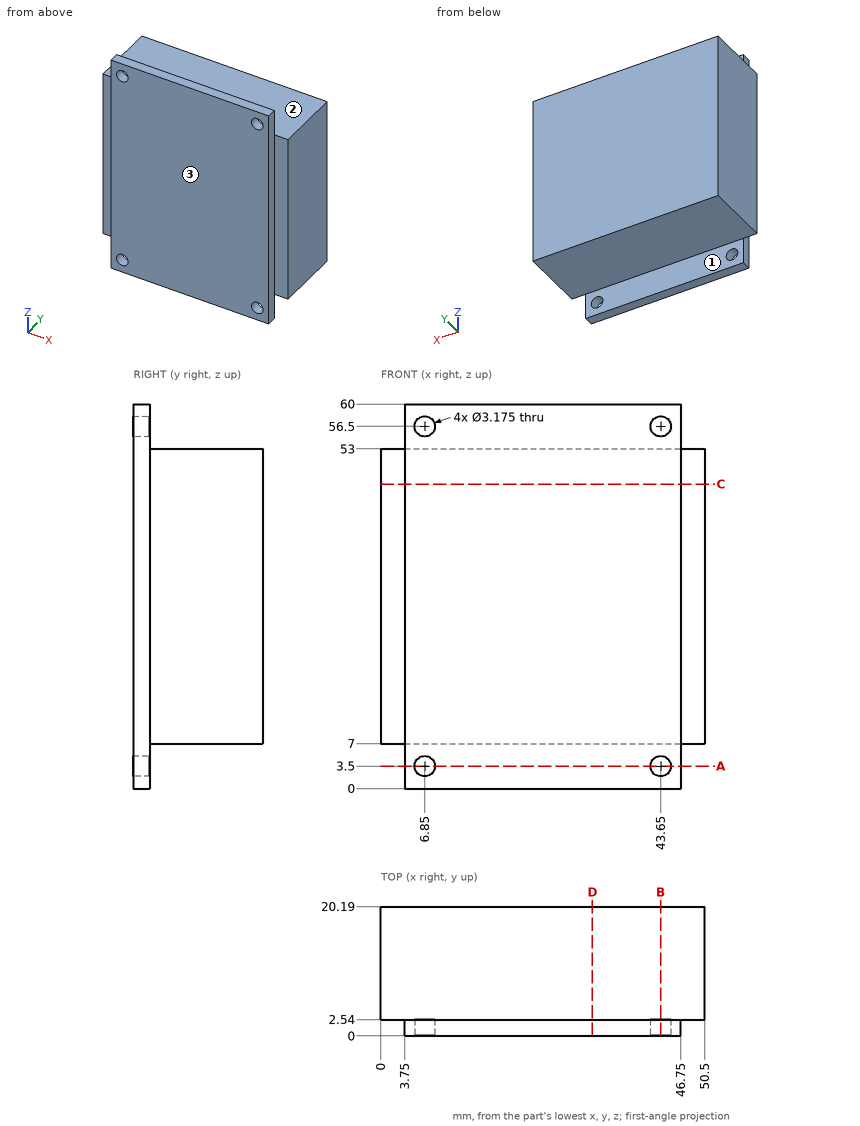
Study the drawing (mm; zero at the part's minimum x, y, z) and answer. A direction names the side the tool comes from. Give positions to 0.01 mm unless a question says otherwise; leave off trailing zeros. Write each loop counter-clockwise with the first axis right and the second up, starting at its lowest first coordinate (ties: lowest second). Pieces come first, ordered by that corner, then holes.
Item 1: Section A-A, the plane z = 3.5 is taken. Write down the section's boundary in (x, y).
Item 2: Which of the six approach directions +Z, -Z, +X, -X, +Y, -Y give full straight-line access (tool end or side, diameter ignored) to the marked faces 1, 2 and 3?
Item 3: Find the intervals of material crossed by line 1 along X through (y, z) = (1.9, 56.5); line 2 along Z through (x, y) = (15.5, 12.25); line 3 along X through (y, z) = (1.5, 20), in increasing order.
Item 4: Section D-D, the plane x = 33 is taken. Write down the section's boundary in (y, z).
Item 5: Section B-B, the plane x = 43.65 is taken. Write down the section's boundary in (y, z), plus the area to 3 significant figures.
Item 6: Flat-ended cylindrical pins translate along their axes: P1, Ø5, axis at y = 10, z = 24, coming from the -X side; P2, Ø1.9, axis at x = 6.85, z = 56.5, coming from the +Y side; P3, Ø5.5, axis at x = 29.5, z = 57.5, coming from the +Y side; P4, Ø8, axis at x = 17.5, y = 17, coming from the +Z side. Find the tip coordinate at first contact, or state that the pin passes through.
Item 7: Section C-C, the plane z = 47.5 is taken. Write down the section's boundary in (x, y), plus the area to 3 significant figures.
Completed:
1. outline: (3.75, 0) - (5.26, 0) - (5.26, 2.54) - (3.75, 2.54) - close; (8.44, 0) - (42.06, 0) - (42.06, 2.54) - (8.44, 2.54) - close; (45.24, 0) - (46.75, 0) - (46.75, 2.54) - (45.24, 2.54) - close
2. face 1: -Z, +X, -X, +Y
2. face 2: +Z, +X, -X, +Y
2. face 3: +Z, -Z, +X, -X, -Y
3. line 1: x = 3.75 to 5.26, 8.44 to 42.06, 45.24 to 46.75
3. line 2: z = 7 to 53
3. line 3: x = 3.75 to 46.75
4. outline: (0, 0) - (2.54, 0) - (2.54, 7) - (20.19, 7) - (20.19, 53) - (2.54, 53) - (2.54, 60) - (0, 60) - close
5. outline: (0, 0) - (2.54, 0) - (2.54, 1.91) - (0, 1.91) - close; (0, 5.09) - (2.54, 5.09) - (2.54, 7) - (20.19, 7) - (20.19, 53) - (2.54, 53) - (2.54, 54.91) - (0, 54.91) - close; (0, 58.09) - (2.54, 58.09) - (2.54, 60) - (0, 60) - close
5. area: 948 mm2
6. P1: stops at x = 0
6. P2: passes through
6. P3: stops at y = 2.54
6. P4: stops at z = 53
7. outline: (0, 2.54) - (3.75, 2.54) - (3.75, 0) - (46.75, 0) - (46.75, 2.54) - (50.5, 2.54) - (50.5, 20.19) - (0, 20.19) - close
7. area: 1,000 mm2
